Study the drawing (mm; zero at the part's minimum x, y, z) and answer. A direction names the side the tool comes from. Give positions to 0.01 mm unless a question says otherwise; leave off trailing zeros. Loops run counter-clockwise (first coordinate to the right, second up) from the corner with the lowest first, then second, coordinate; pieces in that order, holes last. Notation, with made-up numbers: (-8, -28) - (6, -28) arc R22 ccw to (6, 6) - close; hole circle Ø11 at (3, -25). An arc over 180 degrees is marked (long way). Write item = value, one per line. Start each with the question number.
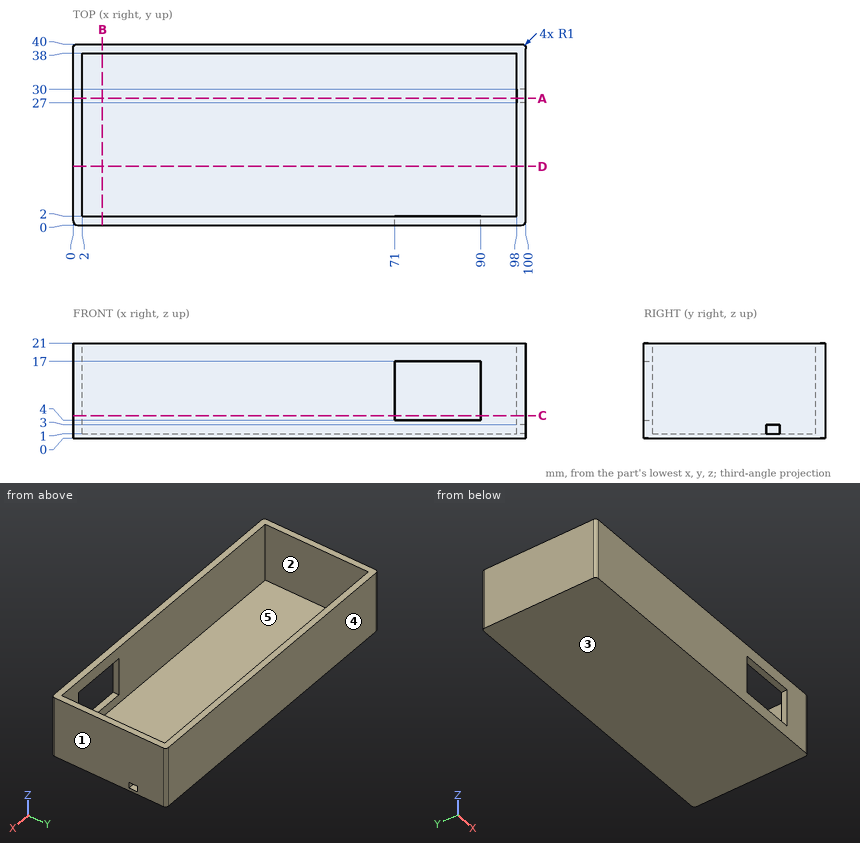
1. Consider line 1 along Y through (x, z) = (48, 4.5); line 2 along X through (y, z) = (32, 15.5); line 3 along Z through (x, y) = (59, 19). Determine where each line is inside the solid, lowest interval first. Write a range as [from, to].
2. A cutting plane is placed at D-D on y = 13. Give the vertices of the cut face in (x, z), and give its area (3 significant figures).
3. A cutting plane is placed at C-C on z = 5. Give the vertices of the cut face in (x, y).
4. Given P1, Ø1, axis at x = 86.5, z = 10.5, coming from the -Y side; P2, Ø1, axis at x = 45, y = 34, coming from the +Z side; P3, Ø0.6, axis at x = 99.5, z = 1.5, coming from the +Y side, each flat-ended and moving along its own axis, determine where each tip first touches the part or whether it passes through.
5. A tool of negligible diameter and unlimited length cuts with its end or side. For the marked faces 1 and 2, from which of +Z, -Z, +X, -X, +Y, -Y can it reach the whole face along a straight path? Write none if from no direction.
6. A cutting plane is placed at A-A on y = 28. Give the vertices of the cut face in (x, z).
7. For a pull along Y with two mould halves and no side action, classify the marked faces 3, 4 and 5 as released by +Y, released by -Y, zero draft, split by the parting line, or undercut.
8. A cutting plane is placed at B-B on x = 6.5. Give the vertices of the cut face in (y, z), and give its area (3 significant figures).
Reply:
q1.line_1 = [0, 2], [38, 40]
q1.line_2 = [0, 2], [98, 100]
q1.line_3 = [0, 1]
q2.outline = (0, 0) - (100, 0) - (100, 21) - (98, 21) - (98, 1) - (2, 1) - (2, 21) - (0, 21) - close
q2.area = 180 mm^2
q3.outline = (0, 1) arc R1 ccw to (1, 0) - (71, 0) - (71, 2) - (2, 2) - (2, 38) - (98, 38) - (98, 2) - (90, 2) - (90, 0) - (99, 0) arc R1 ccw to (100, 1) - (100, 39) arc R1 ccw to (99, 40) - (1, 40) arc R1 ccw to (0, 39) - close
q4.P1 = 38
q4.P2 = 1
q4.P3 = 39.98
q5.face_1 = +Z, -Z, +X, +Y, -Y
q5.face_2 = +Z
q6.outline = (0, 0) - (100, 0) - (100, 1) - (2, 1) - (2, 21) - (0, 21) - close; (98, 3) - (100, 3) - (100, 21) - (98, 21) - close
q7.face_3 = zero draft
q7.face_4 = released by +Y
q7.face_5 = undercut
q8.outline = (0, 0) - (40, 0) - (40, 21) - (38, 21) - (38, 1) - (2, 1) - (2, 21) - (0, 21) - close
q8.area = 120 mm^2
